Geometry: final body of the model. Coordinates: model frame, mm. A direction names the side the tool comes from. Give positions to 0.01 mm unless a question says otherwise; leave off trailing zeros. Write each loop counter-clockwise with the first axis right and the second up, starting at its lowest first coordinate (ties: lowest second). Pieces come first, ordered by that corner, then holes. Notation, with made-up numbers: (24, -21.5) -> (74, -21.5) arc R20 ccw to (74, -7.5) -> close; hole circle Ø10 at (64.25, -30). An arc over 180 degrees is marked (long way). Answer in a Markdown table with one row per item. Add a question column.
Item 1: First-contact query: P1, Ø4.5, axis at x = 0, z = 0, coming from the +Y side; P2, Ø0.9, axis at x = 0.5, y = 4, coming from the -Z side; P3, Ø1.5, axis at x = -51, y = 3, coming from the -Z side. Flat tips, straight axial feed; report the tip coordinate or a pass-through.
Item 2: Section query B-B on x = 0. Output: boundary loops of the cut face in (y, z), plus the area to 3 significant figures.
Item 3: Draft query along X for faces 3 (the cylindrical face through (44.745, 3.972, -44.375)), 4 (the flat face through (16, 0, -1)), 5 (the cylindrical face through (-9.764, 1.479, -74.362)). Return one class per face: +X half, -X half, draft (parallel to the pull), parting line (faces both ways), or undercut.
Item 4: Section query D-D on x = -63. Output: boundary loops of the cut face in (y, z).
Item 5: Material intervals for probe 1 along X at (y, z) = (5.55, -33); probe 2 along Z at (x, y) = (-11.5, 3.95); probe 3 along X at (y, z) = (2.95, -32.5), sorted ascending. Write a range as from..to.
Item 6: Section query A-A on z = 0. Output: boundary loops of the cut face in (x, y).
Item 7: Access query for faces 1 (the cylindrical face through (-44.745, 3.972, 44.375)), 2 (the flat face through (66.3, 3, 27.4)). Directions: +Z, -Z, +X, -X, +Y, -Y. A direction counts if a zero-diameter tool reaches every point of the face in a straight line with its end or side. Return the directions, or none.
Item 8: Section query C-C on z = -56.5. Output: boundary loops of the cut face in (x, y).
```python
from build123d import *

# Parameters (mm, degrees)
SKETCH1_R                    = 75
BOSS_EXTRUDE1_DEPTH          = 3
SKETCH2_R                    = 71.5
BOSS_EXTRUDE2_DEPTH          = 3
SKETCH3_R                    = 2
CUT_EXTRUDE1_DEPTH           = 7
CHAMFER1_SIZE                = 2
CIRPATTERN1_COUNT            = 4
CHAMFER1_OF_CIRPATTERN1_SIZE = 2
SKETCH4_R                    = 2
CUT_EXTRUDE2_DEPTH           = 7
CHAMFER2_SIZE                = 2
CUT_EXTRUDE4_DEPTH           = 3


with BuildPart() as part:
    # Sketch1 → Boss-Extrude1 (new body)
    with BuildSketch(Plane(origin=(0, 0, 0), x_dir=(1, 0, 0), z_dir=(0, 1, 0))):
        Circle(SKETCH1_R)
    extrude(amount=BOSS_EXTRUDE1_DEPTH)

    # Sketch2 → Boss-Extrude2 (add)
    with BuildSketch(Plane(origin=(0, 3, 0), x_dir=(1, 0, 0), z_dir=(0, 1, 0))):
        Circle(SKETCH2_R)
    extrude(amount=BOSS_EXTRUDE2_DEPTH)

    # Sketch3 → Cut-Extrude1 (cut, through all)
    with BuildSketch(Plane.XZ):
        with Locations((45.961940777, 45.961940777)):
            Circle(SKETCH3_R)
    cut_extrude1 = extrude(amount=-CUT_EXTRUDE1_DEPTH, mode=Mode.SUBTRACT)

    # Chamfer1
    chamfer1_edges = [part.edges().sort_by_distance(p)[0] for p in [
        (43.961940777, 0, 45.961940777),
    ]]
    chamfer(chamfer1_edges, length=CHAMFER1_SIZE)

    # CirPattern1: Cut-Extrude1 ×4 about axis
    cirpattern1_axis = Axis((0, 0, 0), (0, 1, 0))
    for i in range(1, CIRPATTERN1_COUNT):
        add(cut_extrude1.rotate(cirpattern1_axis, i * 360 / CIRPATTERN1_COUNT), mode=Mode.SUBTRACT)

    # Chamfer1 of CirPattern1
    chamfer1_of_cirpattern1_edges = [part.edges().sort_by_distance(p)[0] for p in [
        (45.961940777, 0, -43.961940777),
        (-43.961940777, 0, -45.961940777),
        (-45.961940777, 0, 43.961940777),
    ]]
    chamfer(chamfer1_of_cirpattern1_edges, length=CHAMFER1_OF_CIRPATTERN1_SIZE)

    # Sketch4 → Cut-Extrude2 (cut, through all)
    with BuildSketch(Plane.XZ):
        Circle(SKETCH4_R)
    extrude(amount=-CUT_EXTRUDE2_DEPTH, mode=Mode.SUBTRACT)

    # Chamfer2
    chamfer2_edges = [part.edges().sort_by_distance(p)[0] for p in [
        (-2, 0, 0),
    ]]
    chamfer(chamfer2_edges, length=CHAMFER2_SIZE)

    # Sketch5 → Cut-Extrude4 (cut)
    with BuildSketch(Plane(origin=(0, 6, 0), x_dir=(1, 0, 0), z_dir=(0, 1, 0))):
        with BuildLine():
            Line((-10, 70.797245709), (10, 70.797245709))
            ThreePointArc((10, 70.797245709), (0, 71.5), (-10, 70.797245709))
        make_face()
    extrude(amount=-CUT_EXTRUDE4_DEPTH, mode=Mode.SUBTRACT)


solid = part.part
```
Findings below:
| question | item | result |
|---|---|---|
| 1 | P1 | stops at y = 6 |
| 1 | P2 | stops at z = -70.8 |
| 1 | P3 | stops at z = -55.68 |
| 2 | outline | (0, -75) -> (3, -75) -> (3, -70.8) -> (6, -70.8) -> (6, -2) -> (2, -2) -> (0, -4) -> close; (0, 4) -> (2, 2) -> (6, 2) -> (6, 71.5) -> (3, 71.5) -> (3, 75) -> (0, 75) -> close |
| 2 | area | 849 mm^2 |
| 3 | face 3 | undercut |
| 3 | face 4 | draft |
| 3 | face 5 | parting line |
| 4 | outline | (0, -40.69) -> (3, -40.69) -> (3, -33.81) -> (6, -33.81) -> (6, 33.81) -> (3, 33.81) -> (3, 40.69) -> (0, 40.69) -> close |
| 5 | probe 1 | x = -63.43..63.43 |
| 5 | probe 2 | z = -70.57..70.57 |
| 5 | probe 3 | x = -67.59..67.59 |
| 6 | outline | (-75, 0) -> (-4, 0) -> (-2, 2) -> (-2, 6) -> (-71.5, 6) -> (-71.5, 3) -> (-75, 3) -> close; (2, 2) -> (4, 0) -> (75, 0) -> (75, 3) -> (71.5, 3) -> (71.5, 6) -> (2, 6) -> close |
| 7 | face 1 | +Y, -Y |
| 7 | face 2 | +Y |
| 8 | outline | (-49.32, 0) -> (49.32, 0) -> (49.32, 3) -> (43.82, 3) -> (43.82, 6) -> (-43.82, 6) -> (-43.82, 3) -> (-49.32, 3) -> close |
